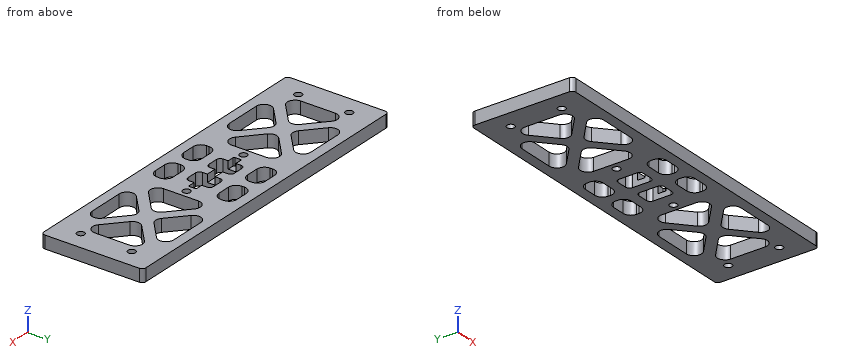
from build123d import *

# Parameters (mm, degrees)
SKETCH_1_W          = 130
SKETCH_1_H          = 40
SKETCH_1_R          = 1.45
EXTRUDE_1_DEPTH     = 5
SKETCH_3_W          = 24
SKETCH_3_H          = 3
CUT_EXTRUDE_1_DEPTH = 3
SKETCH_4_W          = 7
SKETCH_4_H          = 10
CUT_EXTRUDE_2_DEPTH = 69.190908485
SKETCH_5_W          = 11
SKETCH_5_H          = 7
CUT_EXTRUDE_3_DEPTH = 69.190908485
FILLET_1_R          = 3
FILLET_2_R          = 1.5
FILLET_3_R          = 1.5
FILLET_4_R          = 0.5


with BuildPart() as part:
    # 草图1 → 凸台-拉伸1 (new body)
    with BuildSketch(Plane.XY):
        Rectangle(SKETCH_1_W, SKETCH_1_H)
        with Locations((-57.5, -10)):
            Circle(SKETCH_1_R, mode=Mode.SUBTRACT)
        with Locations((-57.5, 10)):
            Circle(SKETCH_1_R, mode=Mode.SUBTRACT)
        with Locations(Location((57.5, -10, 0), (0, 0, 180))):
            Circle(SKETCH_1_R, mode=Mode.SUBTRACT)
        with Locations(Location((57.5, 10, 0), (0, 0, 180))):
            Circle(SKETCH_1_R, mode=Mode.SUBTRACT)
        with Locations((-15, 0)):
            Circle(SKETCH_1_R, mode=Mode.SUBTRACT)
        with Locations((15, 0)):
            Circle(SKETCH_1_R, mode=Mode.SUBTRACT)
    extrude(amount=EXTRUDE_1_DEPTH)

    # 草图3 → 切除-拉伸1 (cut)
    with BuildSketch(Plane.XY.offset(5)):
        Rectangle(SKETCH_3_W, SKETCH_3_H)
    extrude(amount=-CUT_EXTRUDE_1_DEPTH, mode=Mode.SUBTRACT)

    # 草图4 → 切除-拉伸2 (cut, through all)
    with BuildSketch(Plane.XY.offset(5)):
        with Locations((-5.5, 0)):
            Rectangle(SKETCH_4_W, SKETCH_4_H)
        with Locations((5.5, 0)):
            Rectangle(SKETCH_4_W, SKETCH_4_H)
    extrude(amount=-CUT_EXTRUDE_2_DEPTH, mode=Mode.SUBTRACT)

    # 草图5 → 切除-拉伸3 (cut, through all)
    with BuildSketch(Plane.XY.offset(5)):
        Polygon((-51.346241304, 16), (-36.25, 2.668254433), (-21.153758696, 16), align=None)
        Polygon((-54.5, 13.448628684), (-39.271405755, 0), (-54.5, -13.448628684), align=None)
        Polygon((-18, 13.448628684), (-18, -13.448628684), (-33.228594245, 0), align=None)
        Polygon((-51.346241304, -16), (-21.153758696, -16), (-36.25, -2.668254433), align=None)
        with Locations((-7.5, 12.5)):
            Rectangle(SKETCH_5_W, SKETCH_5_H)
        with Locations((-7.5, -12.5)):
            Rectangle(SKETCH_5_W, SKETCH_5_H)
        with Locations((7.5, -12.5)):
            Rectangle(SKETCH_5_W, SKETCH_5_H)
        with Locations((7.5, 12.5)):
            Rectangle(SKETCH_5_W, SKETCH_5_H)
        Polygon((36.25, -2.668254433), (51.346241304, -16), (21.153758696, -16), align=None)
        Polygon((33.228594245, 0), (18, 13.448628684), (18, -13.448628684), align=None)
        Polygon((54.5, -13.448628684), (54.5, 13.448628684), (39.271405755, 0), align=None)
        Polygon((21.153758696, 16), (51.346241304, 16), (36.25, 2.668254433), align=None)
    extrude(amount=-CUT_EXTRUDE_3_DEPTH, mode=Mode.SUBTRACT)

    # 圆角1
    fillet_1_edges = [part.edges().sort_by_distance(p)[0] for p in [
        (-13, -16, 2.5),
        (-13, -9, 2.5),
        (-2, -9, 2.5),
        (-2, -16, 2.5),
        (13, 16, 2.5),
        (13, 9, 2.5),
        (2, 9, 2.5),
        (2, 16, 2.5),
        (2, -9, 2.5),
        (13, -9, 2.5),
        (13, -16, 2.5),
        (2, -16, 2.5),
        (21.153758696, -16, 2.5),
        (36.25, -2.668254433, 2.5),
        (51.346241304, -16, 2.5),
        (-51.346241304, 16, 2.5),
        (-21.153758696, 16, 2.5),
        (-36.25, 2.668254433, 2.5),
        (-2, 16, 2.5),
        (-2, 9, 2.5),
        (-13, 9, 2.5),
        (-13, 16, 2.5),
        (-51.346241304, -16, 2.5),
        (-36.25, -2.668254433, 2.5),
        (-21.153758696, -16, 2.5),
        (-18, -13.448628684, 2.5),
        (-33.228594245, 0, 2.5),
        (-18, 13.448628684, 2.5),
        (36.25, 2.668254433, 2.5),
        (21.153758696, 16, 2.5),
        (51.346241304, 16, 2.5),
        (54.5, -13.448628684, 2.5),
        (39.271405755, 0, 2.5),
        (54.5, 13.448628684, 2.5),
        (33.228594245, 0, 2.5),
        (18, -13.448628684, 2.5),
        (18, 13.448628684, 2.5),
        (-54.5, -13.448628684, 2.5),
        (-54.5, 13.448628684, 2.5),
        (-39.271405755, 0, 2.5),
    ]]
    fillet(fillet_1_edges, radius=FILLET_1_R)

    # 圆角2
    fillet_2_edges = [part.edges().sort_by_distance(p)[0] for p in [
        (-2, 5, 2.5),
        (-9, -5, 2.5),
        (-2, -5, 2.5),
        (-9, 5, 2.5),
        (9, 5, 2.5),
        (2, -5, 2.5),
        (9, -5, 2.5),
        (2, 5, 2.5),
    ]]
    fillet(fillet_2_edges, radius=FILLET_2_R)

    # 圆角3
    fillet_3_edges = [part.edges().sort_by_distance(p)[0] for p in [
        (65, -20, 2.5),
        (-65, -20, 2.5),
        (-65, 20, 2.5),
        (65, 20, 2.5),
    ]]
    fillet(fillet_3_edges, radius=FILLET_3_R)

    # 圆角4
    fillet_4_edges = [part.edges().sort_by_distance(p)[0] for p in [
        (12, 1.5, 3.5),
        (12, -1.5, 3.5),
        (-12, -1.5, 3.5),
        (-12, 1.5, 3.5),
    ]]
    fillet(fillet_4_edges, radius=FILLET_4_R)


solid = part.part
Design review of the part built by this model. Coordinates are the model's own, in mm. Give positions to 0.01 mm unless a question says otherwise; leave off trailing zeros. Order: outer loops, then holes, each group sorted by start corner. A loop starts at its lowest first (then second) coordinate and runs counter-clockwise, first axis right, second up. Notation, with made-up numbers: (27, 19) - (63, 19) arc R31 cw to (63, 47) - close; hole circle Ø8 at (3, -8.5). An arc over 180 degrees is marked (long way). Use CSV: the item, a comma, the result in double quotes. Start each with the question number.
Q1. For line 1 (Y direction, x = 57.5, z = 2.65); line 2 (Y direction, x = 15, z = 2.65); line 3 (X direction, y = -11.5, z = 1.55), list the stretches that pass through material, from the lowest coordinate up.
Q2. Take a section at A-A (x = 15). State the section outline as (y, z) points.
Q3. Take a section at C-C (z = 3.8). Count the separate pieces of the cut face and the enclosed holes in it, and give its area (3 significant figures).
Q4. Take a section at D-D (x = -33). State the section outline as (y, z) points.
Q5. Take a section at B-B (x = 57.5). State the section outline as (y, z) points, and give its area (3 significant figures).
Calculated:
1,line 1,"y = -20 to -11.45, -8.55 to 8.55, 11.45 to 20"
1,line 2,"y = -20 to -1.45, 1.45 to 20"
1,line 3,"x = -65 to -46.02, -26.48 to -12.96, -2.04 to 2.04, 12.96 to 26.48, 46.02 to 65"
2,outline,"(-20, 0) - (-1.45, 0) - (-1.45, 5) - (-20, 5) - close; (1.45, 0) - (20, 0) - (20, 5) - (1.45, 5) - close"
3,separate pieces,"1"
3,enclosed holes,"19"
3,area,"3,290 mm²"
4,outline,"(-20, 0) - (-16, 0) - (-16, 5) - (-20, 5) - close; (-5.54, 0) - (5.54, 0) - (5.54, 5) - (-5.54, 5) - close; (16, 0) - (20, 0) - (20, 5) - (16, 5) - close"
5,outline,"(-20, 0) - (-11.45, 0) - (-11.45, 5) - (-20, 5) - close; (-8.55, 0) - (8.55, 0) - (8.55, 5) - (-8.55, 5) - close; (11.45, 0) - (20, 0) - (20, 5) - (11.45, 5) - close"
5,area,"171 mm²"
